CAD build for the part. Positions are in the model's coordinates, mm. A direction names the side the tool comes from. Give positions to 0.01 mm unless a question says otherwise; leave off trailing zeros. Order: outer loops, then holes, each group sorted by start corner. A loop starts at its lowest first (then second) coordinate and runs counter-clockwise, first axis right, second up. Notation, with made-up numbers: (54.5, 20) -> (77.5, 20) arc R25 ccw to (77.5, 33) -> close; hole circle Ø9 at (3.25, 51). An arc over 180 degrees is marked (long way). Use one line per item in the form item = value. Start each with the question number.
1) Mould opens along Z. For faces 5 (the face through (-3, 6, -3)), 6 (the face through (-6.056, 0.493, 5.069)), 7 (the face through (-9.699, 2.465, 9.715)) say: pulls with the +Z half, pulls with the -Z half, needs draft (parallel to the pull), parting line crosses it, or undercut.
2) Cut at C-C, the plane x = 0. Give the cut face in (y, z).
3) Probe line 1 (Z direction, x = 0, y = 3.6); line 2 (Y direction, x = 0.75, z = 6). List the from-to ranges inside material, lowest first.
4) Drop flat-ended pins along their axis: P1, Ø3.5, axis at x = 0, z = 0, coming from the +Y side; P2, Ø2.5, axis at y = 3, z = -3, coming from the +X side; P3, Ø2.5, axis at x = -1, y = 1.5, coming from the +Z side; P4, Ø3, axis at x = -8.5, z = -3.5, coming from the -Y side. Give the stop position or say it passes through.
5) Cut at D-D, the plane x = -8. Give the cut face in (y, z), and give its area (3 significant figures).
6) Cut at A-A, the plane y = 0.45. Give the cut face in (x, z), and give its area (3 significant figures).
7) Tool access for faces 1 (the face through (0.6, 0.49, -4.74)), 2 (the face through (0, 2, 10)), 3 (the face through (10, 2, 0)), 4 (the face through (9.715, 2.465, 9.699)): list every direction of +Z, -Z, +X, -X, +Y, -Y with a clear straight run to the whole face (end or side of a thin tool).
8) Cut at B-B, the plane z = -6.5. Give the cut face in (x, y).
Autodesk Inventor part; units mm, degrees
ref_plane "YZ Plane" through (0, 0, 0) normal (1, 0, 0) x (0, 1, 0)
ref_plane "XZ Plane" through (0, 0, 0) normal (0, 1, 0) x (-1, 0, 0)
ref_plane "XY Plane" through (0, 0, 0) normal (0, 0, 1) x (1, 0, 0)
sketch "Sketch1" plane through (0, 0, 0) normal (0, 1, 0) x (-1, 0, 0)
  line L0 (9, -10) -> (-9, -10)
  line L1 (-10, -9) -> (-10, 9)
  line L2 (-9, 10) -> (9, 10)
  line L3 (10, 9) -> (10, -9)
  line L4 (10, 10) -> (-10, -10) construction
  line L5 (10, -10) -> (-10, 10) construction
  arc A0 (10, 9) -> (9, 10) centre (9, 9) ccw
  arc A1 (9, -10) -> (10, -9) centre (9, -9) ccw
  arc A2 (-10, -9) -> (-9, -10) centre (-9, -9) ccw
  arc A3 (-9, 10) -> (-10, 9) centre (-9, 9) ccw
  point P0 (0, 0)
  point P1 (0, 0)
  dimension "d7" = 20
  dimension "d9" = 20
  dimension "d10" = 1
extrude "Extrusion1" add sketch "Sketch1" along normal blind 5
sketch "Sketch2" plane through (0, 5, 0) normal (0, 1, 0) x (1, 0, 0)
  line L0 (-10, 9) -> (-10, -9)
  arc A0 (-10, -9) -> (-9, -10) centre (-9, -9) ccw
  line L1 (-9, -10) -> (9, -10)
  arc A1 (9, -10) -> (10, -9) centre (9, -9) ccw
  line L2 (10, -9) -> (10, 9)
  arc A2 (10, 9) -> (9, 10) centre (9, 9) ccw
  line L3 (9, 10) -> (-9, 10)
  arc A3 (-9, 10) -> (-10, 9) centre (-9, 9) ccw
  line L4 (9, -11.5) -> (-9, -11.5)
  arc A4 (-11.5, -9) -> (-9, -11.5) centre (-9, -9) ccw
  line L5 (-11.5, -9) -> (-11.5, 9)
  arc A5 (-9, 11.5) -> (-11.5, 9) centre (-9, 9) ccw
  line L6 (-9, 11.5) -> (9, 11.5)
  arc A6 (11.5, 9) -> (9, 11.5) centre (9, 9) ccw
  line L7 (11.5, 9) -> (11.5, -9)
  arc A7 (9, -11.5) -> (11.5, -9) centre (9, -9) ccw
  circle A8 centre (0, 0) radius 2.75
  dimension "d16" = 1.5
  dimension "d19" = 5.5
extrude "Extrusion3" add sketch "Sketch2" along normal blind 1 contours A3 L3 A2 L2 A1 L1 A0 L0 | L4 A4 L5 A5 L6 A6 L7 A7
sketch "Sketch3" plane through (0, 0, 0) normal (0, -1, 0) x (1, 0, 0)
  line L0 (-8.3335, 1.5979) -> (-1.5979, -8.3335)
  line L1 (-1.5979, -8.3335) -> (-0.3669, -5.7051)
  line L2 (1.9204, -4.6109) -> (3.3678, -4.9657)
  line L3 (3.3678, -4.9657) -> (3.4632, -3.4705)
  line L4 (5.4592, -1.5979) -> (8.3335, -1.5979)
  line L5 (8.3335, -1.5979) -> (1.5979, 8.3335)
  line L6 (1.5979, 8.3335) -> (-1.2764, 8.3335)
  line L7 (-3.2724, 6.4609) -> (-3.3678, 4.9657)
  line L8 (-3.3678, 4.9657) -> (-4.8403, 5.2316)
  line L9 (-6.9654, 4.1955) -> (-8.3335, 1.5979)
  line L10 (-3.3678, 4.9657) -> (3.3678, -4.9657) construction
  arc A0 (-4.8403, 5.2316) -> (-6.9654, 4.1955) centre (-5.1958, 3.2635) ccw
  arc A1 (-1.2764, 8.3335) -> (-3.2724, 6.4609) centre (-1.2764, 6.3335) ccw
  arc A2 (5.4592, -1.5979) -> (3.4632, -3.4705) centre (5.4592, -3.5979) ccw
  arc A3 (1.9204, -4.6109) -> (-0.3669, -5.7051) centre (1.4443, -6.5534) ccw
  line L11 (-4.9657, -3.3678) -> (0, 0) construction
  line L12 (0, 0) -> (4.9657, 3.3678) construction
  line L13 (-2.6449, 7.792) -> (4.0907, -2.1393) construction
  line L14 (-2.7456, 0.156) -> (0.8707, 2.6085) construction
  circle A4 centre (0, 0) radius 2.75 construction
  line L15 (-6.0723, 5.0611) -> (0.5812, -4.7492) construction
  line L16 (-3.0915, 3.7031) -> (2.297, -4.242)
  line L17 (2.297, -4.242) -> (3.0915, -3.7031)
  line L18 (3.0915, -3.7031) -> (-2.297, 4.242)
  line L19 (-2.297, 4.242) -> (-3.0915, 3.7031)
  point P0 (-0.9375, 1.3822)
  point P1 (-2.6942, 3.9725)
  point P2 (2.6942, -3.9725)
  point P3 (-0.3973, -0.2694)
  dimension "d77" = 2
  dimension "d78" = 12
  dimension "d79" = 12
  dimension "d80" = 12
  dimension "d81" = 6
  dimension "d82" = 6
  dimension "d85" = 9.6
  dimension "d86" = 0.96
extrude "Extrusion7" cut sketch "Sketch3" against normal blind 1
extrude "Extrusion8" cut sketch "Sketch2" against normal blind 2 contours A8
equation "\"d7\" = button_side"
equation "\"d9\" = d7"
equation "\"d78\" = d79"
equation "\"d79\" = 0.6 * button_side"
equation "\"d80\" = d79"
equation "\"d81\" = d82"
equation "\"d82\" = 0.5 * d79"
equation "\"d85\" = 0.8 * d80"
equation "\"d86\" = 0.1 * d85"
equation "\"d0\" = 122"
equation "\"d1\" = 77"
equation "\"d4\" = 19"
equation "\"d5\" = 1"
equation "\"d8\" = 25"
equation "\"d13\" = 1.5"
equation "\"d14\" = 0"
equation "\"d15\" = 2"
equation "\"d30\" = 3.1"
equation "\"d31\" = 3"
equation "\"d33\" = 3"
equation "\"d34\" = 2"
equation "\"d36\" = 3"
equation "\"d38\" = 90deg"
equation "\"d39\" = 8"
equation "\"d40\" = 118deg"
equation "\"d44\" = 0"
equation "\"d45\" = 1.2"
equation "\"d46\" = 2"
equation "\"d47\" = 0"
equation "\"d50\" = 25"
equation "\"button_side\" = 20"
equation "\"d3\" = 1.01 * button_side"
equation "\"d2\" = d3"
properties part number "button4" material "Bronze, Soft Tin"
Result:
q1.face_5 = needs draft
q1.face_6 = undercut
q1.face_7 = pulls with the +Z half
q2.outline = (0, -10) -> (5, -10) -> (5, -11.5) -> (6, -11.5) -> (6, -2.75) -> (3, -2.75) -> (3, 2.75) -> (6, 2.75) -> (6, 11.5) -> (5, 11.5) -> (5, 10) -> (0, 10) -> (0, 8.33) -> (1, 8.33) -> (1, 0.86) -> (0, 0.86) -> (0, -0.86) -> (1, -0.86) -> (1, -5.17) -> (0, -5.17) -> close
q3.line_1 = -10 to -2.75, 2.75 to 10
q3.line_2 = 1 to 6
q4.P1 = 3
q4.P2 = 10
q4.P3 = 10
q4.P4 = 0
q5.outline = (0, -10) -> (5, -10) -> (5, -11.5) -> (6, -11.5) -> (6, 11.5) -> (5, 11.5) -> (5, 10) -> (0, 10) -> (0, 2.23) -> (1, 2.23) -> (1, 1.11) -> (0, 1.11) -> close
q5.area = 122 mm²
q6.outline = (-10, -9) arc R1 ccw to (-9, -10) -> (9, -10) arc R1 ccw to (10, -9) -> (10, 9) arc R1 ccw to (9, 10) -> (-9, 10) arc R1 ccw to (-10, 9) -> close; (-3.09, 3.7) -> (2.3, -4.24) -> (3.09, -3.7) -> (-2.3, 4.24) -> close; hole (-8.33, 1.6) -> (-1.6, -8.33) -> (-0.37, -5.71) arc R2 cw to (1.92, -4.61) -> (3.37, -4.97) -> (3.46, -3.47) arc R2 cw to (5.46, -1.6) -> (8.33, -1.6) -> (1.6, 8.33) -> (-1.28, 8.33) arc R2 ccw to (-3.27, 6.46) -> (-3.37, 4.97) -> (-4.84, 5.23) arc R2 ccw to (-6.97, 4.2) -> close
q6.area = 265 mm²
q7.face_1 = -Y
q7.face_2 = +Z, +X, -X, -Y
q7.face_3 = +Z, -Z, +X, -Y
q7.face_4 = +Z, +X, -Y
q8.outline = (-11.5, 5) -> (-10, 5) -> (-10, 0) -> (-2.84, 0) -> (-2.84, 1) -> (-0.74, 1) -> (-0.74, 0) -> (10, 0) -> (10, 5) -> (11.5, 5) -> (11.5, 6) -> (-11.5, 6) -> close
